Autodesk Inventor part; units mm, degrees
ref_plane "YZ Plane" through (0, 0, 0) normal (1, 0, 0) x (0, 1, 0)
ref_plane "XZ Plane" through (0, 0, 0) normal (0, 1, 0) x (-1, 0, 0)
ref_plane "XY Plane" through (0, 0, 0) normal (0, 0, 1) x (1, 0, 0)
sketch "草图1" plane through (0, 0, 0) normal (0, 0, 1) x (1, 0, 0)
  circle A0 centre (0, 0) radius 4
  dimension "d0" = 8
extrude "拉伸1" add sketch "草图1" along normal blind 1
sketch "草图2" plane through (0, 0, 1) normal (0, 0, 1) x (1, 0, 0)
  line L0 (1.4434, -2.5) -> (-1.4434, -2.5)
  line L1 (-1.4434, -2.5) -> (-2.8868, 0)
  line L2 (-2.8868, 0) -> (-1.4434, 2.5)
  line L3 (-1.4434, 2.5) -> (1.4434, 2.5)
  line L4 (1.4434, 2.5) -> (2.8868, 0)
  line L5 (2.8868, 0) -> (1.4434, -2.5)
  line L6 (0, 0) -> (0, 2.5)
  dimension "d3" = 5
extrude "拉伸2" add sketch "草图2" along normal blind 4
sketch "草图3" plane through (0, 0, 0) normal (0, 0, -1) x (-1, 0, 0)
  circle A0 centre (0, 0) radius 2.5
  dimension "d6" = 5
extrude "拉伸3" add sketch "草图3" along normal blind 8
thread "螺纹1"
chamfer "倒角1" distance 0.25 angle 45 1 edges at (2.5, 0, -8)
properties part number "装填斗罩螺丝"
Read the model definition and answer for the solid it produces. Units are mm, in the model's axes. A direction names the side the tool comes from. Coordinates: 2 decimals unless noted, no trailing zeros. Loops run counter-clockwise (first coordinate to the right, second up) from the corner with the lowest first, then second, coordinate; pieces in that order, holes last. Notation, with made-up numbers: (54, -11) -> (60, -11) arc R17 ccw to (60, 18) -> close; hole circle Ø1 at (-23, -9.5). An arc over 180 degrees is marked (long way). Write item = value, one per line. Start each with the question number.
1) Find the intervals of material crossed by L1, parallel to Z at x = -0.75, y = 3.5; L2, parallel to Y at x = -1, z = 3.25; L3, parallel to Y at x = -0.5, z = -4.25, in increasing order. Write a range as from..to.
2) The part is cut by section C-C, the plane y = -3.5. Determine the outline of the cut face in (x, z).
3) Given P1, Ø2.5, axis at x = 0, z = 2.5, coming from the -Y side; P2, Ø4, axis at x = 3, z = -2.5, coming from the +Y side; P3, Ø3, axis at x = 3, y = -3, coming from the +Z side, each flat-ended and moving along its own axis, determine where each tip first touches the part or whether it passes through.
4) The part is cut by section B-B, the plane z = -4.75. Determine the outline of the cut face in (x, y), plus the area to 3 significant figures.
5) For faces 1 (the face through (0, 2.5, 3)), 2 (the face through (2.155, 1.267, 2.972)), 3 (the face through (0, -2.5, 3)), 4 (the face through (-2.155, -1.267, 2.972)), 5 (the face through (2.175, -1.233, 2.972)), determine the directions among +Z, -Z, +X, -X, +Y, -Y from which every point of the face is accessible in a straight line to the end or side of a thin tool.
6) The part is cut by section A-A, the plane x = 0. Determine the outline of the cut face in (y, z), plus the area to 3 significant figures.
Result:
q1.L1 = 0..1
q1.L2 = -2.5..2.5
q1.L3 = -2.45..2.45
q2.outline = (-1.94, 0) -> (1.94, 0) -> (1.94, 1) -> (-1.94, 1) -> close
q3.P1 = -2.5
q3.P2 = 2.29
q3.P3 = 1
q4.outline = circle Ø5 at (0, 0)
q4.area = 19.6 mm²
q5.face_1 = +Z, +X, -X, +Y
q5.face_2 = +Z, +X, +Y
q5.face_3 = +Z, +X, -X, -Y
q5.face_4 = +Z, -X, -Y
q5.face_5 = +Z, +X, -Y
q6.outline = (-4, 0) -> (-2.5, 0) -> (-2.5, -7.75) -> (-2.25, -8) -> (2.25, -8) -> (2.5, -7.75) -> (2.5, 0) -> (4, 0) -> (4, 1) -> (2.5, 1) -> (2.5, 5) -> (-2.5, 5) -> (-2.5, 1) -> (-4, 1) -> close
q6.area = 67.9 mm²
